Design review of the part shown in the three views and the two pictorial views. Dimensions are in mm from the part's minimum x, y and z. Round coordinates to 2 decimals unless told otherwise and drop trailing zeros. Loops run counter-clockwise (first coordinate to the right, second up) from the corner with the lowest first, then second, coordinate; pieces in that order, holes last. Notation, with made-up numbers: (38, 23) -> (82, 23) arc R32 cw to (82, 60) -> close; hole circle Ø2 at (29, 62.25). An arc over 180 degrees is marked (long way). Return JSON: item names as keys, results as strings. Group by question number.
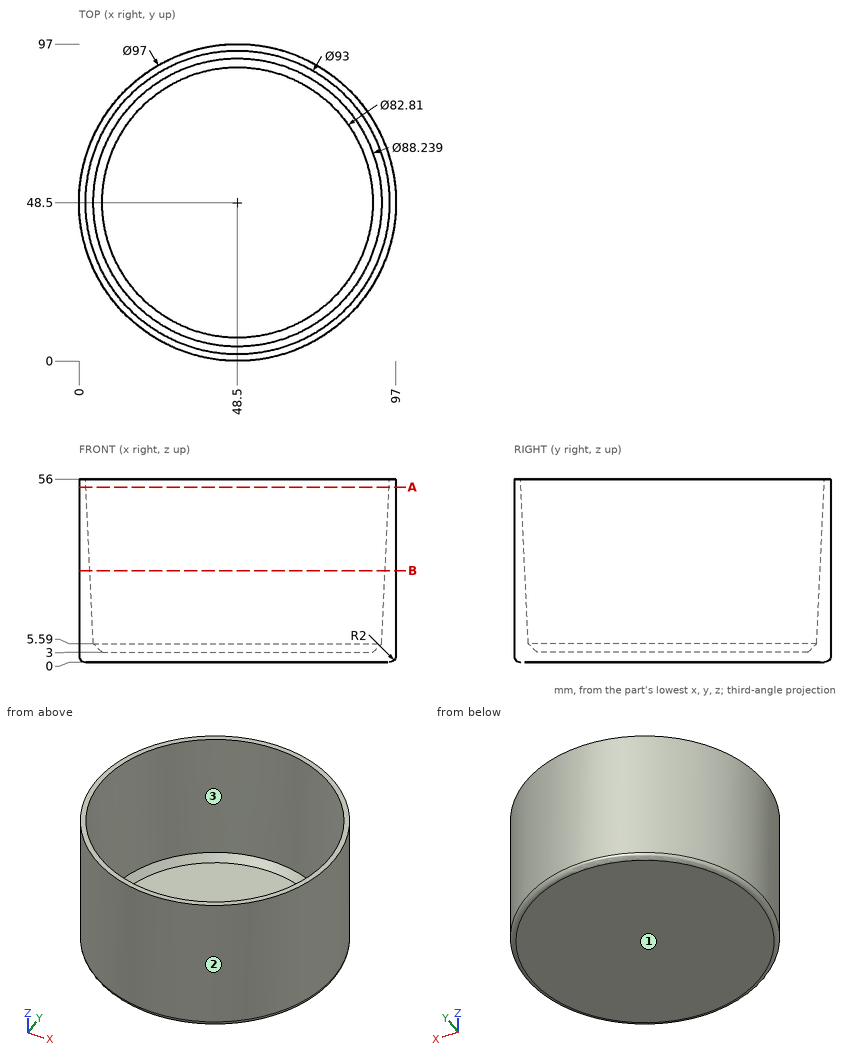
1. We need section B-B, the plane z = 28. Write out the cut boundary in (x, y) (1 decimal).
2. Wall thickness on line 1 (Y direction, x = 18, z = 36); line 2 (X direction, y = 13.5, z = 23.5) (1 decimal); line 3 (Y direction, x = 56, z = 43.5): over which ranges is each line inside the solid? List them lowest first.
3. For P1, Ø8, axis at x = 28.5, z = 12, coming from the +Y side (1 decimal); P2, Ø25, axis at x = 58, y = 61.5, coming from the +Z side; P3, Ø3, axis at x = 74.5, z = 8, coming from the +Y side, all flat-tipped, find the tip position at first contact; note any pin that passes through.
4. We need section A-A, the plane z = 53.5. Write out the cut boundary in (x, y).
5. Draft analysis for pull direction Y (two halves, no side actions). For the marked faces 1, 2 and 3, state which applies: pulls with the +Y half, pulls with the -Y half, needs draft (parallel to the pull), parting line crosses it, or undercut.
Check sheet entries:
{
 "1": {"outline": "circle Ø97 at (48.5, 48.5); hole circle Ø90.4 at (48.5, 48.5)"},
 "2": {"line 1": "y = 10.79 to 14.66, 82.34 to 86.21", "line 2": "x = 14.9 to 20.3, 76.7 to 82.1", "line 3": "y = 0.58 to 3.21, 93.79 to 96.42"},
 "3": {"P1": "stops at y = 94.3", "P2": "stops at z = 3", "P3": "stops at y = 90.36"},
 "4": {"outline": "circle Ø97 at (48.5, 48.5); hole circle Ø92.76 at (48.5, 48.5)"},
 "5": {"face 1": "needs draft", "face 2": "parting line crosses it", "face 3": "undercut"}
}
